Work out the finished part from the listing and answer in its coordinate system (mm). Face numbers are marked on the shaded views. A direction names the side the tool comes from. Give positions to 0.01 mm unless a question says otherwise; leave off trailing zeros. Loops run counter-clockwise (first coordinate to the right, second up) from the corner with the lowest first, then second, coordinate; pieces in that order, holes last. Notation, with made-up numbers: (-39, 12) - (-13, 12) arc R19 ccw to (-13, 18) - close; hole circle Ø3 at (65.5, 35.25). An arc over 180 degrees is marked (long way). Use CSV: the item, a comma, the result in double quotes.
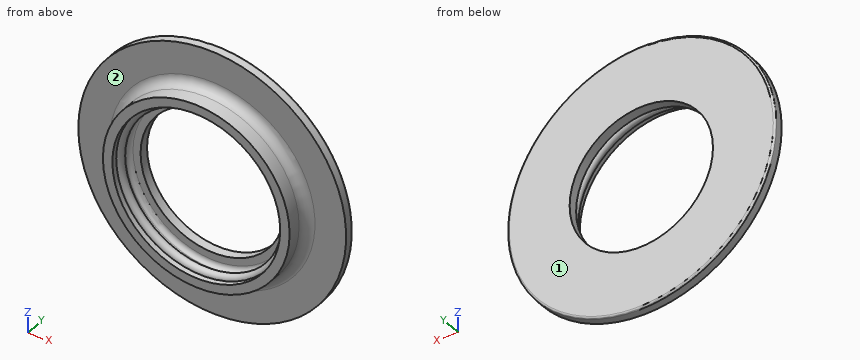
from build123d import *


with BuildPart() as part:
    # Sketch1 → Revolve1 (revolve)
    with BuildSketch(Plane.XY):
        with BuildLine():
            Line((26.42831399, 12.330127019), (26.42831399, 16.330127019))
            ThreePointArc((26.42831399, 16.330127019), (26.721207209, 17.0372338), (27.42831399, 17.330127019))
            Line((27.42831399, 17.330127019), (59.42831399, 17.330127019))
            Line((59.42831399, 17.330127019), (59.42831399, 12.330127019))
            Line((59.42831399, 12.330127019), (55.42831399, 12.330127019))
            ThreePointArc((55.42831399, 12.330127019), (53.660547037, 11.597893972), (52.92831399, 9.830127019))
            Line((52.92831399, 9.830127019), (52.92831399, 8))
            ThreePointArc((52.92831399, 8), (55.42831399, 5.5), (52.92831399, 3))
            Line((52.92831399, 3), (52.92831399, 0))
            Line((52.92831399, 0), (47.92831399, 0))
            Line((47.92831399, 0), (47.92831399, 7.330127019))
            ThreePointArc((47.92831399, 7.330127019), (46.463847896, 10.865660925), (42.92831399, 12.330127019))
            Line((42.92831399, 12.330127019), (26.42831399, 12.330127019))
        make_face()
    revolve(axis=Axis((97.42831399, 39.892585804, 0), (0, -1, 0)))


solid = part.part
Item 1: Given P1, Ø8, axis at y = 6, z = 29, coming from the +X side; P2, Ø5, axis at y = 10.5, z = -32.5, coming from the -X side; P3, Ø1.5, axis at x = 74.5, y = 6.5, coming from the +Z side; P4, Ø25, axis at x = 85, z = -4.5, coming from the -Y side, each flat-ended and moving along its own axis, determine where each tip first touches the part or whether it passes through.
Determined:
P1,"stops at x = 140.15"
P2,"stops at x = 33.46"
P3,"stops at z = 44.25"
P4,"passes through"
Item 2: Find the intervals of material crossed by line 1 (X direction, y = 13.7, z = 0); line 2 (X direction, y = 4.5, z = 18.5); line 3 (Z direction, x = 133, y = 11.25), in increasing order.
Determined:
line 1,"x = 26.43 to 59.43, 135.43 to 168.43"
line 2,"x = 51.52 to 59.49, 135.37 to 143.34"
line 3,"z = -37.1 to -25.99, 25.99 to 37.1"
Item 3: A cutting plane is placed at B-B on y = 5.5. Determine the outline of the cut face in (x, z), and give its area (3 significant figures).
Determined:
outline,"circle Ø99 at (97.43, 0); hole circle Ø84 at (97.43, 0)"
area,"2,160 mm²"
Item 4: A cutting plane is placed at A-A on z = 0. Determine the outline of the cut face in (x, y).
Determined:
outline,"(26.43, 12.33) - (42.93, 12.33) arc R5 cw to (47.93, 7.33) - (47.93, 0) - (52.93, 0) - (52.93, 3) arc R2.5 ccw to (52.93, 8) - (52.93, 9.83) arc R2.5 cw to (55.43, 12.33) - (59.43, 12.33) - (59.43, 17.33) - (27.43, 17.33) arc R1 ccw to (26.43, 16.33) - close; (135.43, 12.33) - (139.43, 12.33) arc R2.5 cw to (141.93, 9.83) - (141.93, 8) arc R2.5 ccw to (141.93, 3) - (141.93, 0) - (146.93, 0) - (146.93, 7.33) arc R5 cw to (151.93, 12.33) - (168.43, 12.33) - (168.43, 16.33) arc R1 ccw to (167.43, 17.33) - (135.43, 17.33) - close"
Item 5: For the marked faces 1 and 2, determine the directions among +Z, -Z, +X, -X, +Y, -Y from which every point of the face is accessible in a straight line to the end or side of a thin tool.
Determined:
face 1,"+Z, -Z, +X, -X, +Y"
face 2,"-Y"
